Autodesk Inventor part; units mm, degrees
ref_plane "Work Plane1" through (-29.1, -14.5, 2.4) normal (0, 0, -1) x (0, 1, 0)
ref_plane "Work Plane2" through (-13.8999, -10.5497, 2.25) normal (0, 0, -1) x (0, 1, 0)
ref_plane "YZ Plane" through (0, 0, 0) normal (1, 0, 0) x (0, 1, 0)
ref_plane "Work Plane1" through (-29.1, -14.5, 2.4) normal (0, 0, -1) x (0, 1, 0)
ref_plane "Work Plane2" through (-13.8999, -10.5497, 2.25) normal (0, 0, -1) x (0, 1, 0)
sketch "Sketch1" plane through (0, 0, 0) normal (0, 0, 1) x (1, 0, 0)
  line L0 (-34.86, 0) -> (34.86, 0) construction
  line L1 (0, -34.86) -> (0, 34.86) construction
  line L2 (0, 0) -> (11.1575, 11.1575) construction
  line L3 (0, 0) -> (15.7791, 0) construction
  line L4 (0, 24.9) -> (16.8009, 24.9)
  line L5 (16.8009, 24.9) -> (16.8009, 21.2415)
  line L6 (16.8009, 21.2415) -> (19.0212, 19.0212)
  line L7 (24.9, 0) -> (24.9, 16.8009)
  line L8 (24.9, 16.8009) -> (21.2415, 16.8009)
  line L9 (21.2415, 16.8009) -> (19.0212, 19.0212)
  line L10 (0, -24.9) -> (16.8009, -24.9)
  line L11 (16.8009, -24.9) -> (16.8009, -21.2415)
  line L12 (16.8009, -21.2415) -> (19.0212, -19.0212)
  line L13 (24.9, 0) -> (24.9, -16.8009)
  line L14 (24.9, -16.8009) -> (21.2415, -16.8009)
  line L15 (21.2415, -16.8009) -> (19.0212, -19.0212)
  line L16 (0, 24.9) -> (-16.8009, 24.9)
  line L17 (-16.8009, 24.9) -> (-16.8009, 21.2415)
  line L18 (-16.8009, 21.2415) -> (-19.0212, 19.0212)
  line L19 (-24.9, 16.8009) -> (-21.2415, 16.8009)
  line L20 (-21.2415, 16.8009) -> (-19.0212, 19.0212)
  line L21 (0, -24.9) -> (-16.8009, -24.9)
  line L22 (-16.8009, -24.9) -> (-16.8009, -21.2415)
  line L23 (-16.8009, -21.2415) -> (-19.0212, -19.0212)
  line L24 (-21.2415, -16.8009) -> (-19.0212, -19.0212)
  line L25 (-24.9, -16.8009) -> (-21.2415, -16.8009)
  line L26 (-24.9, 0) -> (-24.9, -16.8009)
  line L27 (-24.9, 0) -> (-24.9, 16.8009)
  circle A0 centre (0, 0) radius 10
  dimension "d0" = 45
  dimension "d2" = 24.9
  dimension "d3" = 3.14
  dimension "d4" = 26.9
  dimension "d5" = 20
extrude "Extrusion1" add sketch "Sketch1" along normal up to surface (2.25 mm away)
sketch "Sketch5" plane through (0, 0, 0) normal (0, 0, -1) x (-1, 0, 0)
  circle A0 centre (-9.7, 10) radius 1.4
  circle A1 centre (-9.7, -10) radius 1.4
  circle A2 centre (13.8, 0) radius 1.4
  circle A3 centre (-10, 6.9) radius 0.75
  circle A4 centre (10, 6.9) radius 1.25
  point P0 (0, 0)
hole "Hole1" at (-13.8, 0, 0) at (9.7, -10, 0) at (-10, 6.9, 0) at (9.7, 10, 0) direction (0, 0, 1) diameter 3.3 depth 12 tip angle 118
properties part number "20_Cube_insert_Sample_holder"
Part model, mm, in its own coordinate system. A direction names the side the tool comes from. Give positions to 0.01 mm unless a question says otherwise; leave off trailing zeros. Order: outer loops, then holes, each group sorted by start corner. A loop starts at its lowest first (then second) coordinate and runs counter-clockwise, first axis right, second up. Notation, with made-up numbers: (13, -24.75) - (67, -24.75) arc R33 ccw to (67, 8.25) - close; hole circle Ø2 at (-27.75, 44.25). An arc over 180 degrees is marked (long way). Use a Markdown table: item, result.
1) 3-axis set-ups, long thin cutter, end or side, ignore diameter. For faces 4 (the cylindrical face through (8.064, -10.215, 1.141)), 5 (the flat face through (23, 16.801, 1)), 6 (the flat face through (23, -16.801, 1)): which of +Z, -Z, +X, -X, +Y, -Y reach the whole face in a straight line?
Checked values:
| item | result |
|---|---|
| face 4 | +Z, -Z |
| face 5 | +Z, -Z, +X, +Y |
| face 6 | +Z, -Z, +X, -Y |
2) Flat gauge pins, fed straight in: P1, Ø0.7, axis at y = 22, z = 1.5, coming from the -X side; P2, Ø1.1, axis at y = 24, z = 1.5, coming from the +X side; P3, Ø0.7, axis at x = -22.5, z = 1, coming from the +Y side. Where does each tip first touch, or does it go through?
Checked values:
| item | result |
|---|---|
| P1 | x = -16.8 |
| P2 | x = 16.8 |
| P3 | y = 16.8 |
3) Two-plate mould, pull along Y, no slides. Class faces 1 (the flat face through (-16.801, -23, 1)), 2 (the flat face through (-18.99, 19.05, 1.11)), 3 (the cylindrical face through (8.064, 9.785, 1.141)): +Y half, -Y half, draft (parallel to the pull), parting line (faces both ways), or undercut.
Checked values:
| item | result |
|---|---|
| face 1 | draft |
| face 2 | +Y half |
| face 3 | undercut |
4) Saw through at C-C on y = -11. List the corners of the cut face in (x, z).
Checked values:
| item | result |
|---|---|
| outline | (-24.9, 0) - (8.39, 0) - (8.39, 2.25) - (-24.9, 2.25) - close; (11.01, 0) - (24.9, 0) - (24.9, 2.25) - (11.01, 2.25) - close |
5) Probe L1, parallel to X at y = 6.9, z = 0.6; L2, parallel to Y at x = -5.5, z = 0.3; L3, parallel to Y at x = -13.8, z = 0.85. List the from-to ranges inside material, lowest first. Write a range as from..to.
Checked values:
| item | result |
|---|---|
| L1 | -24.9..-11.65, -8.35..-7.24, 7.24..24.9 |
| L2 | -24.9..-8.35, 8.35..24.9 |
| L3 | -24.9..-1.65, 1.65..24.9 |
6) Saw through at D-D on x = -9. List the corners of the cut face in (y, z).
Checked values:
| item | result |
|---|---|
| outline | (-24.9, 0) - (-4.36, 0) - (-4.36, 2.25) - (-24.9, 2.25) - close; (4.36, 0) - (5.59, 0) - (5.59, 2.25) - (4.36, 2.25) - close; (8.21, 0) - (24.9, 0) - (24.9, 2.25) - (8.21, 2.25) - close |
7) Saw through at A-A on x = 0. List the corners of the cut face in (y, z).
Checked values:
| item | result |
|---|---|
| outline | (-24.9, 0) - (-10, 0) - (-10, 2.25) - (-24.9, 2.25) - close; (10, 0) - (24.9, 0) - (24.9, 2.25) - (10, 2.25) - close |
8) Saw through at B-B on z = 1.9. List the corners of the cut face in (x, y), plus the area to 3 significant figures.
Checked values:
| item | result |
|---|---|
| outline | (-24.9, -16.8) - (-21.24, -16.8) - (-16.8, -21.24) - (-16.8, -24.9) - (16.8, -24.9) - (16.8, -21.24) - (21.24, -16.8) - (24.9, -16.8) - (24.9, 16.8) - (21.24, 16.8) - (16.8, 21.24) - (16.8, 24.9) - (-16.8, 24.9) - (-16.8, 21.24) - (-21.24, 16.8) - (-24.9, 16.8) - close; hole circle Ø3.3 at (-13.8, 0); hole circle Ø3.3 at (-10, 6.9); hole circle Ø20 at (0, 0); hole circle Ø3.3 at (9.7, -10); hole circle Ø3.3 at (9.7, 10) |
| area | 1,910 mm² |
